Work out the finished part from the listing and answer in its coordinate system (mm). Face numbers are marked on the shaded views. Coordinates: 2 decimals unless noted, no trailing zeros. Order: outer loops, then holes, each group sorted by start corner. A loop starts at its lowest first (then second) coordinate and runs counter-clockwise, first axis right, second up. Notation, with made-up numbers: (44, 31.25) -> (57, 31.25) arc R33 cw to (57, 65.25) -> close; hole circle Ø10 at (6.25, 51.25). An arc over 180 degrees is marked (long way). Write item = value, one per line. Start each with the question number.
Q1. Straight lines are drawn through the part: L1, parallel to Z at x = 8.15, y = 0; L2, parallel to Z at x = 8.3, y = 1.5; L3, parallel to Y at x = 8.15, z = -5.5. For each, find the intervals that lie inside material, in ascending order. Write a range as from..to.
Q2. The part is cut by section C-C, the plane x = 7.7. Determine the outline of the cut face in (y, z).
Q3. A flat-ended cylindrical pin translates along its axis: pin 1 (1 mm diameter, centred on x = 8, y = 3.5, fed in from -Z). Find the tip coordinate at first contact, or state that the pin passes through.
Q4. The part is cut by section A-A, the plane y = 0. Determine the outline of the cut face in (x, z), plus the area to 3 significant figures.
Q5. For a pull along Z with two mould halves and no side action, classify the marked faces 1, 2 and 3 as +Z half, -Z half, draft (parallel to the pull), parting line (faces both ways), or undercut.
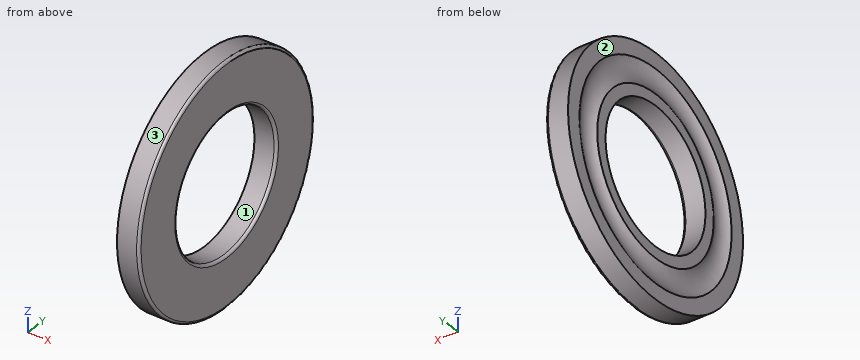
Autodesk Inventor part; units mm, degrees
ref_plane "YZ Plane" through (0, 0, 0) normal (1, 0, 0) x (0, 1, 0)
ref_plane "XZ Plane" through (0, 0, 0) normal (0, 1, 0) x (-1, 0, 0)
ref_plane "XY Plane" through (0, 0, 0) normal (0, 0, 1) x (1, 0, 0)
sketch "Sketch_1" plane through (0, 0, 0) normal (0, 0, 1) x (1, 0, 0)
  line L0 (8.7, 0) -> (6.4048, 0)
  line L1 (6.4048, 9.3214) -> (6.4048, 8)
  line L2 (6.4048, 8) -> (8.7, 8)
  arc A0 (8.7, 8) -> (9, 8.3) centre (8.7, 8.3) ccw
  line L3 (9, 8.3) -> (9, 13.7)
  arc A1 (9, 13.7) -> (8.7, 14) centre (8.7, 13.7) ccw
  line L4 (8.7, 14) -> (6.4048, 14)
  line L5 (6.4048, 14) -> (6.4048, 12.1786)
  arc A2 (6.4048, 9.3214) -> (6.4048, 12.1786) centre (4.5, 10.75) ccw
revolve "Revolution1" add sketch "Sketch_1" angle 360 about axis through (8.7, 0, 0) along (1, 0, 0)
properties part number "SKF_51102_PART3"
Model answer:
q1.L1 = -14..-8, 8..14
q1.L2 = -13.92..-7.86, 7.86..13.92
q1.L3 = -12.87..-5.81, 5.81..12.87
q2.outline = circle Ø28 at (0, 0); hole circle Ø16 at (0, 0)
q3.pin_1 = -13.67
q4.outline = (6.4, -14) -> (8.7, -14) arc R0.3 ccw to (9, -13.7) -> (9, -8.3) arc R0.3 ccw to (8.7, -8) -> (6.4, -8) -> (6.4, -9.32) arc R2.38 cw to (6.4, -12.18) -> close; (6.4, 8) -> (8.7, 8) arc R0.3 ccw to (9, 8.3) -> (9, 13.7) arc R0.3 ccw to (8.7, 14) -> (6.4, 14) -> (6.4, 12.18) arc R2.38 cw to (6.4, 9.32) -> close
q4.area = 29.2 mm2
q5.face_1 = undercut
q5.face_2 = draft
q5.face_3 = parting line
